Autodesk Inventor part; units mm, degrees
ref_plane "YZ Plane" through (0, 0, 0) normal (1, 0, 0) x (0, 1, 0)
ref_plane "XZ Plane" through (0, 0, 0) normal (0, 1, 0) x (-1, 0, 0)
ref_plane "XY Plane" through (0, 0, 0) normal (0, 0, 1) x (1, 0, 0)
sketch "Sketch1" plane through (0, 0, 0) normal (0, 1, 0) x (-1, 0, 0)
  line L0 (7.5, 12.5) -> (-7.5, 12.5)
  line L1 (-7.5, 12.5) -> (-7.5, -12.5)
  line L2 (-7.5, -12.5) -> (7.5, -12.5)
  line L3 (7.5, -12.5) -> (7.5, 12.5)
  line L4 (7.5, 12.5) -> (-7.5, -12.5) construction
  line L5 (-7.5, 12.5) -> (7.5, -12.5) construction
  point P0 (0, 0)
  dimension "d0" = 15
  dimension "d1" = 25
extrude "Extrusion1" add sketch "Sketch1" along normal blind 5
sketch "Sketch2" plane through (0, 5, 0) normal (0, 1, 0) x (1, 0, 0)
  line L0 (-7.5, -12.5) -> (7.5, -12.5)
  line L1 (-7.5, 12.5) -> (-7.5, -12.5)
  line L2 (7.5, 7.5) -> (-7.5, 7.5)
  line L3 (-7.5, 7.5) -> (-7.5, -7.5)
  line L4 (-7.5, -7.5) -> (7.5, -7.5)
  line L5 (7.5, -7.5) -> (7.5, 7.5)
  line L6 (7.5, 7.5) -> (-7.5, -7.5) construction
  line L7 (-7.5, 7.5) -> (7.5, -7.5) construction
  point P0 (0, 0)
  dimension "d5" = 15
extrude "Extrusion2" add sketch "Sketch2" along normal blind 50
sketch "Sketch3" plane through (7.5, 0, 12.5) normal (1, 0, 0) x (0, 0, -1)
  circle A0 centre (12.5, 47.5) radius 5.5
  point P0 (12.5, 0)
  point P1 (14.5, 47.5)
  dimension "d9" = 11
extrude "Extrusion3" cut sketch "Sketch3" against normal blind 13
fillet "Fillet1" radius 7.5 2 edges at (0, 55, -7.5) (0, 55, 7.5)
sketch "Sketch5" plane through (0, 5, 0) normal (0, 1, 0) x (1, 0, 0)
  line L0 (7.5, -7.5) -> (-7.5, -7.5)
  line L1 (-7.5, -12.5) -> (7.5, -12.5)
  line L2 (-7.5, 7.5) -> (7.5, 7.5)
  line L3 (7.5, 12.5) -> (-7.5, 12.5)
  point P0 (0, 0)
  point P1 (0, -10.5)
  point P2 (0, 10.5)
hole "Hole2" at (0, 5, 10.5) at (0, 5, -10.5) direction (0, -1, 0) diameter 3.5 end through all
sketch "Sketch6" plane through (0, 5, 0) normal (0, 1, 0) x (1, 0, 0)
  point P0 (0, 0)
sketch "Sketch8" plane through (0, 5, 0) normal (0, 1, 0) x (1, 0, 0)
  line L0 (-7.5, 12.5) -> (-7.5, 7.5)
  line L1 (7.5, 12.5) -> (-7.5, 12.5)
  line L2 (-7.5, 7.5) -> (7.5, 7.5)
  line L3 (7.5, 7.5) -> (7.5, 12.5)
  line L4 (7.5, 12.5) -> (-7.5, 12.5)
  line L5 (-7.5, 12.5) -> (-7.5, 7.5)
  point P0 (0, 0)
extrude "Extrusion5" cut sketch "Sketch8" against normal through all
properties part number "Holder_slim_1_fod_venstre"
Can you work these out from the model? Positions are in its coordinate system, mm. A direction names the side the tool comes from. Coordinates: 2 decimals unless noted, no trailing zeros. Write each loop counter-clockwise with the first axis right and the second up, starting at its lowest first coordinate (ties: lowest second). Pieces come first, ordered by that corner, then holes. Notation, with made-up numbers: (60, -32.5) -> (105, -32.5) arc R16 ccw to (105, -10.5) -> close; hole circle Ø7 at (80.5, 86). An arc over 180 degrees is marked (long way). Write each question's results on one line, items separated by ' | '. Start each with the question number.
Q1. Imagine slicing it at A-A (x = 0). State how many separate pieces and enclosed holes the cut face has, then the cut area to 3 significant figures.
Q2. Imagine slicing it at D-D (y = 12.5). Write out the boundary of the cut face in (x, z).
Q3. Imagine slicing it at B-B (z = 10.5). Write out the boundary of the cut face in (x, y), then the cut area to 3 significant figures.
Q4. We'd pull the mould along Z, two halves only. Please class faces 4 (the face through (-7.5, 27, 0)), 5 (the face through (0.105, 52.861, 5.245)), 6 (the face through (-0.526, 2.465, 12.169)): +Z half, -Z half, draft (parallel to the pull), parting line (faces both ways), or undercut.
Q5. On a 3-axis mill with a long thin cutter (end or side, diameter ignored), from which of +Z, -Z, +X, -X, +Y, -Y can I reach the whole of each face in a straight line? I mean faces 1 (the face through (-0.105, 52.861, -5.245)), 2 (the face through (-5.5, 48, 0)), 3 (the face through (2, 5, 10)). Say none if no direction works.
Q6. I'm going to push flat-ended pins straight in: pin 1 (6 mm diameter, centred on x = -1, z = 1.5, fed in from -Y); pin 2 (1.5 mm diameter, centred on x = 4, y = 37, fed in from +Z); pin 3 (4 mm diameter, centred on x = 0, z = 10.5, fed in from +Y); pin 4 (3.5 mm diameter, centred on y = 48.5, z = -1.5, fed in from +X). Where does each tip first touch, or does it pass through?
Q7. If I drill on probe 1 along Z at (x, y) = (0, 4.05); probe 2 along Y at (x, z) = (4.25, 0.25); probe 3 along Z at (x, y) = (-5.75, 13.5), over which ranges is the centre line in solid material (lowest first)?
Taken from the geometry:
1) separate pieces: 2 | enclosed holes: 1 | area: 713 mm^2
2) outline: (-7.5, -7.5) -> (7.5, -7.5) -> (7.5, 7.5) -> (-7.5, 7.5) -> close
3) outline: (-7.5, 0) -> (-1.75, 0) -> (-1.75, 5) -> (-7.5, 5) -> close; (1.75, 0) -> (7.5, 0) -> (7.5, 5) -> (1.75, 5) -> close | area: 57.5 mm^2
4) face 4: draft | face 5: +Z half | face 6: undercut
5) face 1: -Z, +X, -X, +Y | face 2: +X | face 3: +Z, +X, -X, +Y
6) pin 1: stops at y = 0 | pin 2: stops at z = 7.5 | pin 3: stops at y = 5 | pin 4: stops at x = -5.5
7) probe 1: z = -7.5 to 8.75, 12.25 to 12.5 | probe 2: y = 0 to 42.01, 52.99 to 55 | probe 3: z = -7.5 to 7.5
